from build123d import *

# Parameters (mm, degrees)
SKETCH1_W           = 25.4
SKETCH1_H           = 25.4
BOSS_EXTRUDE1_DEPTH = 3.175


with BuildPart() as part:
    # Sketch1 → Boss-Extrude1 (new body)
    with BuildSketch(Plane(origin=(0, 0, 0), x_dir=(1, 0, 0), z_dir=(0, 1, 0))):
        Polygon((123.19, 116.586), (123.19, 143.256), (0, 143.256), (0, 116.586), (-3.175, 116.586), (-3.175, 97.536), (0, 97.536), (0, 80.2386), (5.08, 80.2386), (5.08, 82.45475), (7.858125, 82.45475), (7.858125, 80.2386), (9.525, 80.2386), (9.525, 76.7334), (7.858125, 76.7334), (7.858125, 74.51725), (5.08, 74.51725), (5.08, 76.7334), (0, 76.7334), (0, 59.436), (-3.175, 59.436), (-3.175, 40.386), (0, 40.386), (0, 0), (123.19, 0), (123.19, 40.386), (126.365, 40.386), (126.365, 59.436), (123.19, 59.436), (123.19, 76.7334), (118.11, 76.7334), (118.11, 74.51725), (115.331875, 74.51725), (115.331875, 76.7334), (113.665, 76.7334), (113.665, 80.2386), (115.331875, 80.2386), (115.331875, 82.45475), (118.11, 82.45475), (118.11, 80.2386), (123.19, 80.2386), (123.19, 97.536), (126.365, 97.536), (126.365, 116.586), align=None)
        with Locations((61.595, 115.316)):
            Rectangle(SKETCH1_W, SKETCH1_H, mode=Mode.SUBTRACT)
    extrude(amount=BOSS_EXTRUDE1_DEPTH)


solid = part.part
Work out the finished part from the listing and answer in its coordinate system (mm). A direction names the side the tool comes from. Coordinates: 2 decimals unless noted, no trailing zeros. Loops run counter-clockwise (first coordinate to the right, second up) from the corner with the lowest first, then second, coordinate; pieces in that order, holes last. Notation, with made-up numbers: M -33,-15.5 L -11,-15.5 A26 ccw -11,20.5 Z; hole C 62.5,-26.75 d8. An arc over 180 degrees is marked long. Answer in a Markdown table with one row per item. Add a question column.
1. A tool of negligible diameter and unlimited length cuts with its end or side. For faces 5 (the flat face through (3, 2, -76.733)), 6 (the flat face through (123.19, 2, -89)), 7 (the flat face through (48.895, 2, -115)), 8 (the flat face through (123.19, 2, -20)), from which of +Z, -Z, +X, -X, +Y, -Y can it reach the whole face along a straight path? Write none if from no direction.
2. The mould has two halves that part along Z. Classify faces 1 (the flat face through (61, 2, 0)), 2 (the flat face through (61, 2, -128.016)), 3 (the flat face through (61, 0, -73)), 4 (the flat face through (61, 2, -102.616)): pulls with the +Z half, pulls with the -Z half, needs draft (parallel to the pull), parting line crosses it, or undercut.
3. Find section B-B, the plane z = -120. Write down the section's boundary in (x, y) (3 decimals).
4. Consider L1, parallel to X at y = 2.15, z = -123 (3 decimals); L2, parallel to X at y = 0.85, z = -105.5 (3 decimals); L3, parallel to X at y = 2.3, z = -87.5. Determine where each line is inside the solid, lowest interval first.
5. Find section C-C, the plane z = -32. Write down the section's boundary in (x, y) (3 decimals).
6. Find section A-A, the plane x = 59.5. Write down the section's boundary in (y, z) (3 decimals).
7. Flat-ended cylindrical pins translate along their axes: P1, Ø1.6, axis at y = 1, z = -10.5, coming from the -X side; P2, Ø0.7, axis at y = 2, z = -75, coming from the +X side. Find the tip coordinate at first contact, or state that the pin passes through.
Reported:
| question | item | result |
|---|---|---|
| 1 | face 5 | -X, +Y, -Y |
| 1 | face 6 | +X, +Y, -Y |
| 1 | face 7 | +Y, -Y |
| 1 | face 8 | +Z, +X, +Y, -Y |
| 2 | face 1 | pulls with the +Z half |
| 2 | face 2 | undercut |
| 2 | face 3 | needs draft |
| 2 | face 4 | undercut |
| 3 | outline | M 0,0 L 48.895,0 L 48.895,3.175 L 0,3.175 Z; M 74.295,0 L 123.19,0 L 123.19,3.175 L 74.295,3.175 Z |
| 4 | L1 | x = 0 to 48.895, 74.295 to 123.19 |
| 4 | L2 | x = -3.175 to 48.895, 74.295 to 126.365 |
| 4 | L3 | x = 0 to 123.19 |
| 5 | outline | M 0,0 L 123.19,0 L 123.19,3.175 L 0,3.175 Z |
| 6 | outline | M 0,-143.256 L 3.175,-143.256 L 3.175,-128.016 L 0,-128.016 Z; M 0,-102.616 L 3.175,-102.616 L 3.175,0 L 0,0 Z |
| 7 | P1 | stops at x = 0 |
| 7 | P2 | stops at x = 123.19 |
